```python
from build123d import *

# Parameters (mm, degrees)
SKETCH2_W                   = 350
SKETCH2_H                   = 450
BOSS_EXTRUDE1_DEPTH         = 3
CUT_EXTRUDE1_DEPTH          = 3
CHAMFER1_SIZE               = 3
SKETCH4_R                   = 4
CUT_EXTRUDE2_DEPTH          = 3
MIRROR1_OUTLINE_R           = 4
MIRROR1_DEPTH               = 3
MIRROR3_OUTLINE_R           = 4
MIRROR3_DEPTH               = 3
TAP_DRILL_FOR_M5X0_8_TAP1_D = 4.2
M4_CLEARANCE_HOLE1_D        = 4.5


# Read off the part's stored shape, not the designer's step: Mirror1, Mirror3
with BuildPart() as part:
    # Sketch2 → Boss-Extrude1 (new body)
    with BuildSketch(Plane(origin=(0, 0, 0), x_dir=(1, 0, 0), z_dir=(0, 1, 0))):
        Rectangle(SKETCH2_W, SKETCH2_H)
    extrude(amount=BOSS_EXTRUDE1_DEPTH)

    # Sketch3 → Cut-Extrude1 (cut)
    with BuildSketch(Plane(origin=(0, 3, 0), x_dir=(1, 0, 0), z_dir=(0, 1, 0))):
        with BuildLine():
            Line((146, 225), (146, 216))
            Line((146, 216), (157.5, 216))
            Line((157.5, 216), (157.5, 205))
            ThreePointArc((157.5, 205), (162, 200.5), (166.5, 205))
            Line((166.5, 205), (166.5, 210))
            Line((166.5, 210), (175, 210))
            Line((175, 210), (175, 225))
            Line((175, 225), (146, 225))
        make_face()
    extrude(amount=-CUT_EXTRUDE1_DEPTH, mode=Mode.SUBTRACT)

    # Chamfer1
    chamfer1_edges = [part.edges().sort_by_distance(p)[0] for p in [
        (146, 1.5, -225),
        (175, 1.5, -210),
    ]]
    chamfer(chamfer1_edges, length=CHAMFER1_SIZE)

    # Sketch4 → Cut-Extrude2 (cut)
    with BuildSketch(Plane(origin=(0, 3, 0), x_dir=(1, 0, 0), z_dir=(0, 1, 0))):
        with Locations(Location((143, 205, 0), (0, 0, 270))):
            Circle(SKETCH4_R)
        with Locations(Location((162, 185, 0), (0, 0, 270))):
            Circle(SKETCH4_R)
    extrude(amount=-CUT_EXTRUDE2_DEPTH, mode=Mode.SUBTRACT)

    # Mirror1 outline → Mirror1 (cut)
    with BuildSketch(Plane(origin=(0, 0, 0), x_dir=(1, 0, 0), z_dir=(0, 1, 0))):
        with BuildLine():
            Line((-175, 210), (-166.5, 210))
            Line((-166.5, 210), (-166.5, 205))
            ThreePointArc((-166.5, 205), (-162, 200.5), (-157.5, 205))
            Line((-157.5, 205), (-157.5, 216))
            Line((-157.5, 216), (-146, 216))
            Line((-146, 216), (-146, 222))
            Line((-146, 222), (-143, 225))
            Line((-143, 225), (-175, 225))
            Line((-175, 225), (-175, 210))
        make_face()
        with Locations((-162, 185)):
            Circle(MIRROR1_OUTLINE_R)
        with Locations((-143, 205)):
            Circle(MIRROR1_OUTLINE_R)
    extrude(amount=MIRROR1_DEPTH, mode=Mode.SUBTRACT)

    # Mirror3 outline → Mirror3 (cut)
    with BuildSketch(Plane(origin=(0, 0, 0), x_dir=(1, 0, 0), z_dir=(0, 1, 0))):
        with BuildLine():
            Line((172, -210), (166.5, -210))
            Line((166.5, -210), (166.5, -205))
            ThreePointArc((166.5, -205), (162, -200.5), (157.5, -205))
            Line((157.5, -205), (157.5, -216))
            Line((157.5, -216), (146, -216))
            Line((146, -216), (146, -222))
            Line((146, -222), (143, -225))
            Line((143, -225), (175, -225))
            Line((175, -225), (175, -207))
            Line((175, -207), (172, -210))
        make_face()
        with BuildLine():
            Line((-175, -225), (-143, -225))
            Line((-143, -225), (-146, -222))
            Line((-146, -222), (-146, -216))
            Line((-146, -216), (-157.5, -216))
            Line((-157.5, -216), (-157.5, -205))
            ThreePointArc((-157.5, -205), (-162, -200.5), (-166.5, -205))
            Line((-166.5, -205), (-166.5, -210))
            Line((-166.5, -210), (-172, -210))
            Line((-172, -210), (-175, -207))
            Line((-175, -207), (-175, -225))
        make_face()
        with Locations((-143, -205)):
            Circle(MIRROR3_OUTLINE_R)
        with Locations((143, -205)):
            Circle(MIRROR3_OUTLINE_R)
        with Locations((-162, -185)):
            Circle(MIRROR3_OUTLINE_R)
        with Locations((162, -185)):
            Circle(MIRROR3_OUTLINE_R)
    extrude(amount=MIRROR3_DEPTH, mode=Mode.SUBTRACT)

    # Tap Drill for M5x0.8 Tap1 (through all)
    with Locations(Plane(origin=(0, 3, 0), x_dir=(1, 0, 0), z_dir=(0, 1, 0))):
        with Locations((-147.15, 12.5), (-26.45, 12.5), (-26.45, -162.5), (-147.15, -162.5), (-137.5, 162.15), (-167.5, 177.15), (-167.5, 147.15), (137.5, 162.15), (167.5, 177.15), (167.5, 147.15), (-147.15, -87.5), (-26.45, -62.5), (-45.833333333, 162.15), (45.833333333, 162.15)):
            Hole(TAP_DRILL_FOR_M5X0_8_TAP1_D / 2)

    # M4 Clearance Hole1 (through all)
    with Locations(Plane(origin=(0, 3, 0), x_dir=(1, 0, 0), z_dir=(0, 1, 0))):
        with Locations((90, -0.5), (135, -33.5), (135, -183.5), (90, -150.5)):
            Hole(M4_CLEARANCE_HOLE1_D / 2)


solid = part.part
```
Geometry check sheet. Reference: the model listing, model coordinates, mm. Coordinates: 2 decimals unless noted, no trailing zeros. Answer as a JSON object with one key per item and string values. Group by question number.
Item 1: Scan lines: probe 1 along Z at (x, y) = (-167.5, 1.05); probe 2 along X at (y, z) = (1.5, 162.5); probe 3 along Z at (x, y) = (-26.45, 0.8). Record each from-to range of solid material in increasing order.
Item 2: Sectioned sample at A-A, the plane y = 0.75. Give the number of separate pieces and of enclosed holes in the cut face, and give its area (3 significant figures).
Item 3: Depth check by flat-ended pin: pin 1 Ø0.9 at (x, y) = (153.5, 2) entering from +Z; pin 2 Ø1.5 at (y, z) = (2, -211) entering from -X. Enter the tip coordinate at first touch or a pass-through.
Resolved:
{
 "1": {"probe 1": "-210 to -179.25, -175.05 to -149.25, -145.05 to 210", "probe 2": "-175 to -149.25, -145.05 to -28.55, -24.35 to 175", "probe 3": "-225 to -14.6, -10.4 to 60.4, 64.6 to 160.4, 164.6 to 225"},
 "2": {"separate pieces": "1", "enclosed holes": "26", "area": "155,000 mm^2"},
 "3": {"pin 1": "z = 216", "pin 2": "x = -157.5"}
}
